The listing builds one solid part. Answer for the finished solid, in the listing's coordinates (mm). Round coordinates to 2 decimals unless told otherwise and drop trailing zeros. Loops run counter-clockwise (first coordinate to the right, second up) from the corner with the lowest first, then second, coordinate; pieces in that order, holes last. Notation, with made-up numbers: M 55,74 L 106,74 A14 ccw 106,95 Z; hole C 6.25,70 d9. An arc over 180 degrees is marked long. Answer as a JSON object with one key per item and string values.
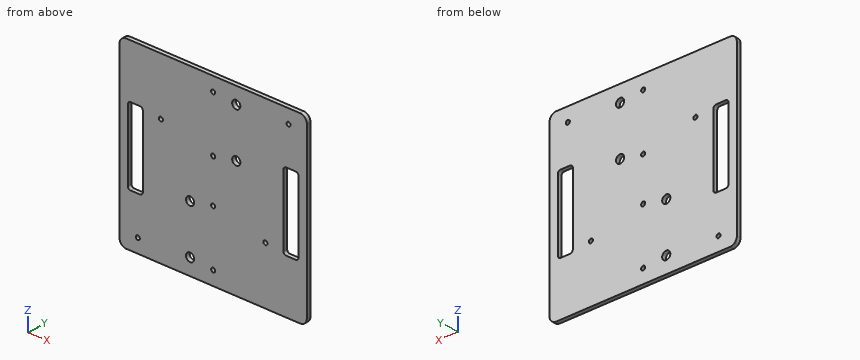
```python
from build123d import *

# Parameters (mm, degrees)
SKETCH1_W                = 138
SKETCH1_H                = 131
BOSS_EXTRUDE1_DEPTH      = 3
SKETCH2_R                = 3
SKETCH2_R_2              = 1.5
SKETCH2_W                = 11
SKETCH2_H                = 55
CUT_EXTRUDE1_DEPTH       = 4
FILLET1_R                = 5
FILLET2_R                = 2
CIRPATTERN1_COUNT        = 2
FILLET2_OF_CIRPATTERN1_R = 2


with BuildPart() as part:
    # Sketch1 → Boss-Extrude1 (new body)
    with BuildSketch(Plane(origin=(0, 0, 0), x_dir=(1, 0, 0), z_dir=(0, 1, 0))):
        Rectangle(SKETCH1_W, SKETCH1_H)
    extrude(amount=BOSS_EXTRUDE1_DEPTH)

    # Sketch2 → Cut-Extrude1 (cut, through all)
    with BuildSketch(Plane(origin=(0, 3, 0), x_dir=(1, 0, 0), z_dir=(0, 1, 0))):
        with Locations((-17, 18.7)):
            Circle(SKETCH2_R)
        with Locations((-17, 53.7)):
            Circle(SKETCH2_R)
        with Locations((0, 55.5)):
            Circle(SKETCH2_R_2)
        with Locations((0, 15.5)):
            Circle(SKETCH2_R_2)
        with Locations((-55.5, 55.5)):
            Circle(SKETCH2_R_2)
        with Locations((-38.5, -24.5)):
            Circle(SKETCH2_R_2)
        with Locations((-57.3, 0.5)):
            Rectangle(SKETCH2_W, SKETCH2_H)
    cut_extrude1 = extrude(amount=-CUT_EXTRUDE1_DEPTH, mode=Mode.SUBTRACT)

    # Fillet1
    fillet1_edges = [part.edges().sort_by_distance(p)[0] for p in [
        (-69, 1.5, -65.5),
        (69, 1.5, -65.5),
        (69, 1.5, 65.5),
        (-69, 1.5, 65.5),
    ]]
    fillet(fillet1_edges, radius=FILLET1_R)

    # Fillet2
    fillet2_edges = [part.edges().sort_by_distance(p)[0] for p in [
        (-51.8, 1.5, -28),
        (-51.8, 1.5, 27),
        (-62.8, 1.5, 27),
        (-62.8, 1.5, -28),
    ]]
    fillet(fillet2_edges, radius=FILLET2_R)

    # CirPattern1: Cut-Extrude1 ×2 about axis
    cirpattern1_axis = Axis((0, 0, 0), (0, 1, 0))
    for i in range(1, CIRPATTERN1_COUNT):
        add(cut_extrude1.rotate(cirpattern1_axis, i * 360 / CIRPATTERN1_COUNT), mode=Mode.SUBTRACT)

    # Fillet2 of CirPattern1
    fillet2_of_cirpattern1_edges = [part.edges().sort_by_distance(p)[0] for p in [
        (51.8, 1.5, 28),
        (51.8, 1.5, -27),
        (62.8, 1.5, -27),
        (62.8, 1.5, 28),
    ]]
    fillet(fillet2_of_cirpattern1_edges, radius=FILLET2_OF_CIRPATTERN1_R)


solid = part.part
```
Item 1: The part is cut by section A-A (z = 18.7). Give the vertices of the cut face in (x, y), then the cut area to 3 significant figures.
Values follow:
{"outline": "M -69,0 L -62.8,0 L -62.8,3 L -69,3 Z; M -51.8,0 L 14,0 L 14,3 L -51.8,3 Z; M 20,0 L 51.8,0 L 51.8,3 L 20,3 Z; M 62.8,0 L 69,0 L 69,3 L 62.8,3 Z", "area": "330 mm^2"}
Item 2: Straight lines are drawn through the part: line 1 (X direction, y = 2.6, z = 8.5); line 2 (Z direction, x = 0, y = 0.8); line 3 (Z direction, x = -17, y = 1.05). For each, find the intervals that lie inside material, in ascending order.
Values follow:
{"line 1": "-69 to -62.8, -51.8 to 51.8, 62.8 to 69", "line 2": "-65.5 to -57, -54 to -17, -14 to 14, 17 to 54, 57 to 65.5", "line 3": "-65.5 to -56.7, -50.7 to -21.7, -15.7 to 65.5"}
Item 3: The part is cut by section B-B (y = 1.4). Give the number of separate pieces and of enclosed holes in the cut face, then the cut area to 3 significant figures.
Values follow:
{"separate pieces": "1", "enclosed holes": "14", "area": "16,700 mm^2"}
Item 4: Flat-ended cylindrical pins translate along their axes: P1, Ø5, axis at x = -55.5, z = -55.5, coming from the -Y side; P2, Ø2.5, axis at x = -38.5, z = 24.5, coming from the +Y side. Find the tip coordinate at first contact, or state that the pin passes through.
Values follow:
{"P1": "y = 0", "P2": "through"}
